Could you check a few things on this model? Use its own coordinates, in mm. A direction names the side the tool comes from. Coordinates: 2 decimals unless noted, no trailing zeros. Write each loop counter-clockwise with the first axis right and the second up, starting at its lowest first coordinate (ties: lowest second). Pieces come first, ordered by that corner, then holes. Notation, with made-up numbers: M -22.5,-4.75 L 29.5,-4.75 A26 cw 29.5,15.25 Z; hole C 23,51 d5. An arc over 180 degrees is marked long. Answer as CSV lines item,"result". Start each with the question number.
Item 1: I'm going to push a flat-ended pin straight in: P1, Ø3, axis at x = -23.75, z = -32.5, coming from the -Y side. Where does the tip first touch, or does it pass through?
Item 2: Suppose I cut it at C-C, the plane x = -7.5. Write out the boundary of the cut face in (y, z), and give its area (3 significant figures).
Item 3: If I drill on line 1 along Z through (x, y) = (-23.75, -0.95); line 2 along X through (y, z) = (0.3, -32.5); line 3 along X through (y, z) = (-0.8, 5.5), over which ranges is the centre line in solid material (lowest first)? Write a range as [from, to].
Item 4: We'd pull the mould along X, two halves only. Please class faces 3 (the flat face through (-35, 0, 0)), 4 (the flat face through (0, 0, 35)), 5 (the flat face through (30, 0, 0)): +X half, -X half, draft (parallel to the pull), parting line (faces both ways), or undercut.
Item 5: Suppose I cut it at A-A, the plane x = 23.75. Write out the boundary of the cut face in (y, z).
Item 6: On a 3-axis mill with a long thin cutter (end or side, diameter ignored), from which of +Z, -Z, +X, -X, +Y, -Y can I reach the whole of each face in a straight line? I mean faces 1 (the flat face through (0, 2.5, 31)), 2 (the flat face through (0, 0, 30)). Say none if no direction works.
Item 7: Suppose I cut it at B-B, the plane z = 32.5. Write out the boundary of the cut face in (x, y), and give its area (3 significant figures).
Item 8: Suppose I cut it at D-D, the plane z = -7. Write out the boundary of the cut face in (x, y).
```python
from build123d import *

# Parameters (mm, degrees)
SKETCH1_W           = 70
SKETCH1_H           = 70
SKETCH1_R           = 1.6
SKETCH1_W_2         = 60
SKETCH1_H_2         = 60
BOSS_EXTRUDE1_DEPTH = 2.5


with BuildPart() as part:
    # Sketch1 → Boss-Extrude1 (new body, symmetric)
    with BuildSketch(Plane(origin=(0, 0, 0), x_dir=(1, 0, 0), z_dir=(0, 1, 0))):
        Rectangle(SKETCH1_W, SKETCH1_H)
        with Locations((-23.75, 32.5)):
            Circle(SKETCH1_R, mode=Mode.SUBTRACT)
        with Locations((23.75, 32.5)):
            Circle(SKETCH1_R, mode=Mode.SUBTRACT)
        with Locations((23.75, -32.5)):
            Circle(SKETCH1_R, mode=Mode.SUBTRACT)
        with Locations((-23.75, -32.5)):
            Circle(SKETCH1_R, mode=Mode.SUBTRACT)
        Rectangle(SKETCH1_W_2, SKETCH1_H_2, mode=Mode.SUBTRACT)
    extrude(amount=BOSS_EXTRUDE1_DEPTH, both=True)


solid = part.part
```
Ans:
1,P1,"passes through"
2,outline,"M -2.5,-35 L 2.5,-35 L 2.5,-30 L -2.5,-30 Z; M -2.5,30 L 2.5,30 L 2.5,35 L -2.5,35 Z"
2,area,"50.0 mm^2"
3,line 1,"z = [-35, -34.1], [-30.9, -30], [30, 30.9], [34.1, 35]"
3,line 2,"x = [-35, -25.35], [-22.15, 22.15], [25.35, 35]"
3,line 3,"x = [-35, -30], [30, 35]"
4,face 3,"-X half"
4,face 4,"draft"
4,face 5,"undercut"
5,outline,"M -2.5,-35 L 2.5,-35 L 2.5,-34.1 L -2.5,-34.1 Z; M -2.5,-30.9 L 2.5,-30.9 L 2.5,-30 L -2.5,-30 Z; M -2.5,30 L 2.5,30 L 2.5,30.9 L -2.5,30.9 Z; M -2.5,34.1 L 2.5,34.1 L 2.5,35 L -2.5,35 Z"
6,face 1,"+Z, -Z, +X, -X, +Y"
6,face 2,"+Y, -Y"
7,outline,"M -35,-2.5 L -25.35,-2.5 L -25.35,2.5 L -35,2.5 Z; M -22.15,-2.5 L 22.15,-2.5 L 22.15,2.5 L -22.15,2.5 Z; M 25.35,-2.5 L 35,-2.5 L 35,2.5 L 25.35,2.5 Z"
7,area,"318 mm^2"
8,outline,"M -35,-2.5 L -30,-2.5 L -30,2.5 L -35,2.5 Z; M 30,-2.5 L 35,-2.5 L 35,2.5 L 30,2.5 Z"
